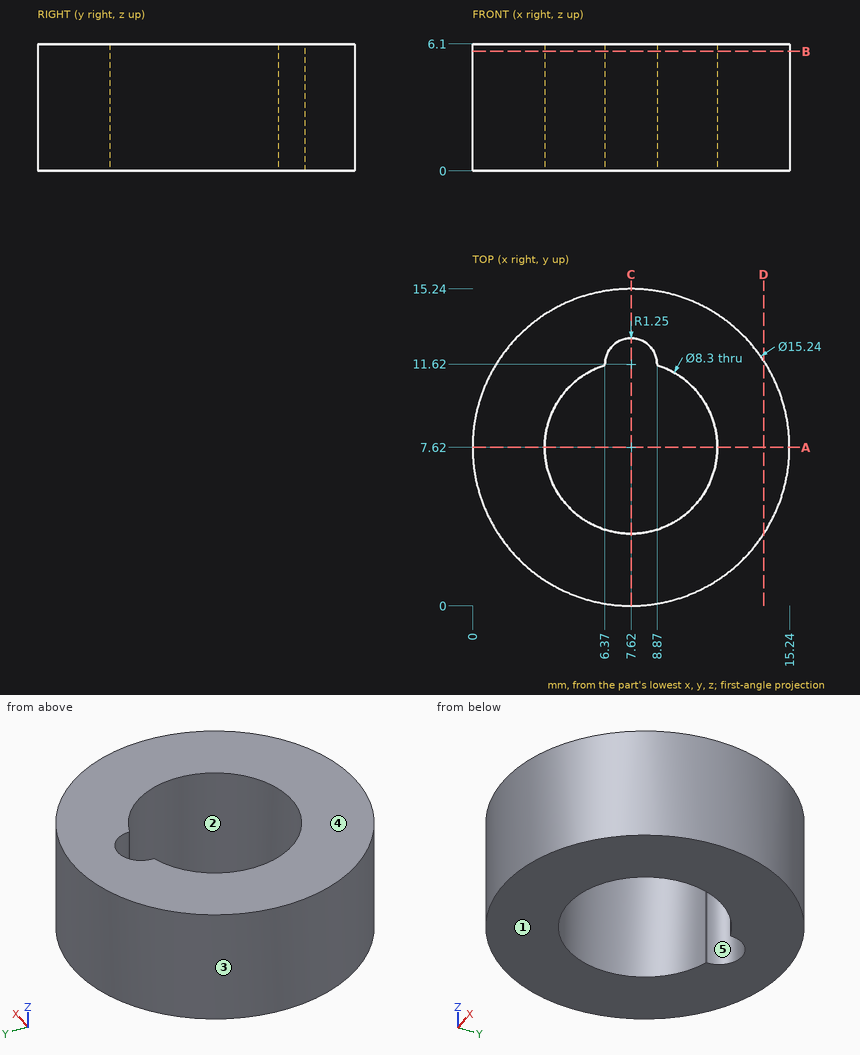
Study the drawing (mm; zero at the part's minimum x, y, z) and answer. A direction names the side the tool comes from. Give positions to 0.01 mm unless a question says otherwise; leave off trailing zeros. Order: outer loops, then holes, each group sorted by start corner. A loop starts at its lowest first (then second) coordinate and runs counter-clockwise, first axis right, second up. Notation, with made-up numbers: (-8.5, -7) - (26.5, -7) arc R32 cw to (26.5, 32) - close; hole circle Ø9 at (50.5, 41.5). An arc over 180 degrees is marked (long way). Use one line per item in the form item = value. Start each with the question number.
(1) For the marked faces 4 and 5, determine the directions among +Z, -Z, +X, -X, +Y, -Y from which every point of the face is accessible in a straight line to the end or side of a thin tool.
(2) A cutting plane is placed at D-D, the plane x = 14. Write down the section's boundary in (y, z).
(3) A cutting plane is placed at C-C, the plane x = 7.62. Write down the section's boundary in (y, z).
(4) The mould has two halves that part along Y. Classify the marked faces 1, 2 and 3: released by +Y, released by -Y, zero draft, split by the parting line, or undercut.
(5) A cutting plane is placed at A-A, the plane y = 7.62. Write down the section's boundary in (x, z).
(6) Flat-ended cylindrical pins translate along their axes: pin 1 Ø1.5 at (x, z) = (12.5, 1) entering from +Y; pin 2 Ø1.5 at (x, z) = (4, 3.5) entering from -Y; pin 3 Ø1 at (x, z) = (1.5, 1.5) entering from -Y. Find the tip coordinate at first contact, or state that the pin passes through.
(7) Consider line 1 (Y direction, x = 11.25, z = 3); line 2 (X direction, y = 5.75, z = 3.5); line 3 (X direction, y = 5.25, z = 0.75). Determine where each line is inside the solid, lowest interval first. Write a range as from..to.
(8) A cutting plane is placed at B-B, the plane z = 5.75. Write down the section's boundary in (x, y).
Ans:
q1.face_4 = +Z, +X, -X, +Y, -Y
q1.face_5 = +Z, -Z
q2.outline = (3.45, 0) - (11.79, 0) - (11.79, 6.1) - (3.45, 6.1) - close
q3.outline = (0, 0) - (3.47, 0) - (3.47, 6.1) - (0, 6.1) - close; (12.87, 0) - (15.24, 0) - (15.24, 6.1) - (12.87, 6.1) - close
q4.face_1 = zero draft
q4.face_2 = undercut
q4.face_3 = split by the parting line
q5.outline = (0, 0) - (3.47, 0) - (3.47, 6.1) - (0, 6.1) - close; (11.77, 0) - (15.24, 0) - (15.24, 6.1) - (11.77, 6.1) - close
q6.pin_1 = 14.02
q6.pin_2 = 0.56
q6.pin_3 = 2.47
q7.line_1 = 0.92..5.61, 9.63..14.32
q7.line_2 = 0.23..3.92, 11.32..15.01
q7.line_3 = 0.38..4.21, 11.03..14.86
q8.outline = circle Ø15.24 at (7.62, 7.62); hole (6.37, 11.58) arc R4.15 ccw (long way) to (8.87, 11.58) - (8.87, 11.62) arc R1.25 ccw to (6.37, 11.62) - close
